```python
from build123d import *

# Parameters (mm, degrees)
BOSS_EXTRUDE1_DEPTH      = 38.1
CUT_EXTRUDE1_DEPTH       = 48.641761051
F_5_16_CLEARANCE_HOLE1_D = 8.3312
FILLET1_R                = 3.175
FILLET2_R                = 6.35


with BuildPart() as part:
    # Sketch1 → Boss-Extrude1 (new body)
    with BuildSketch(Plane.XY.offset(19.05)):
        with BuildLine():
            Line((0, 38.1), (0, 0))
            Line((0, 0), (14.986, 0))
            Line((14.986, 0), (14.986, -35.0266))
            ThreePointArc((14.986, -35.0266), (19.476128061, -33.166728061), (21.336, -28.6766))
            Line((21.336, -28.6766), (21.336, 6.35))
            Line((21.336, 6.35), (6.35, 6.35))
            Line((6.35, 6.35), (6.35, 31.75))
            ThreePointArc((6.35, 31.75), (4.490128061, 36.240128061), (0, 38.1))
        make_face()
    extrude(amount=-BOSS_EXTRUDE1_DEPTH)

    # Sketch2 → Cut-Extrude1 (cut, through all)
    with BuildSketch(Plane.ZY):
        with BuildLine():
            Line((-4.1656, 29.3624), (-4.1656, 16.6624))
            ThreePointArc((-4.1656, 16.6624), (0, 12.4968), (4.1656, 16.6624))
            Line((4.1656, 16.6624), (4.1656, 29.3624))
            ThreePointArc((4.1656, 29.3624), (0, 33.528), (-4.1656, 29.3624))
        make_face()
    extrude(amount=-CUT_EXTRUDE1_DEPTH, mode=Mode.SUBTRACT)

    # 5/16 Clearance Hole1 (through all)
    with Locations(Plane.ZY.offset(-14.986)):
        with Locations((0, -19.05)):
            Hole(F_5_16_CLEARANCE_HOLE1_D / 2)

    # Fillet1
    fillet1_edges = [part.edges().sort_by_distance(p)[0] for p in [
        (14.986, 0, 0),
    ]]
    fillet(fillet1_edges, radius=FILLET1_R)

    # Fillet2
    fillet2_edges = [part.edges().sort_by_distance(p)[0] for p in [
        (6.35, 6.35, 0),
        (21.336, 6.35, 0),
    ]]
    fillet(fillet2_edges, radius=FILLET2_R)


solid = part.part
```
Work out the finished part from the listing and answer in its coordinate system (mm). A direction names the side the tool comes from. Give positions to 0.01 mm unless a question says otherwise; leave off trailing zeros. Write each loop counter-clockwise with the first axis right and the second up, starting at its lowest first coordinate (ties: lowest second). Pieces come first, ordered by that corner, then holes.
(1) Which of the six approach directions +Z, -Z, +X, -X, +Y, -Y give full straight-line access (tool end or side, diameter ignored) to faces 1 (the flat face through (3, 23, 4.166)), 2 (the flat face through (6.35, 22, 12)), 3 (the flat face through (14.986, -19, 5))?
Final values:
face 1: +X, -X
face 2: +Z, -Z, +X, +Y
face 3: +Z, -Z, -X, -Y
(2) Straight lines are drawn through the part: line 1 (Z direction, x = 2.25, y = 22); line 2 (X direction, y = 18, z = -9.5); line 3 (Y direction, x = 20, z = 0). For each, find the intervals that lie inside material, in ascending order.
Final values:
line 1: z = -19.05 to -4.17, 4.17 to 19.05
line 2: x = 0 to 6.35
line 3: y = -32.57 to -23.22, -14.88 to 3.9
(3) The part is cut by section B-B on z = -9.5. Write down the section's boundary in (x, y) (3 decimals), plus the area to 3 significant figures.
Final values:
outline: (0, 0) - (11.811, 0) arc R3.175 cw to (14.986, -3.175) - (14.986, -35.027) arc R6.35 ccw to (21.336, -28.677) - (21.336, 0) arc R6.35 ccw to (14.986, 6.35) - (12.7, 6.35) arc R6.35 cw to (6.35, 12.7) - (6.35, 31.75) arc R6.35 ccw to (0, 38.1) - close
area: 544 mm2
(4) The mould has two halves that part along Z. Classify faces 4 (the flat face through (21.336, -14.5, 0.3)), 5 (the flat face through (3, 23, -4.166)): pulls with the +Z half, pulls with the -Z half, needs draft (parallel to the pull), parting line crosses it, or undercut.
Final values:
face 4: needs draft
face 5: undercut
(5) The part is cut by section C-C on z = 2. Write down the section's boundary in (x, y) (3 decimals).
Final values:
outline: (0, 0) - (11.811, 0) arc R3.175 cw to (14.986, -3.175) - (14.986, -15.396) - (21.336, -15.396) - (21.336, 0) arc R6.35 ccw to (14.986, 6.35) - (12.7, 6.35) arc R6.35 cw to (6.35, 12.7) - (6.35, 13.008) - (0, 13.008) - close; (0, 33.016) - (6.222, 33.016) arc R6.35 ccw to (0, 38.1) - close; (14.986, -35.027) arc R6.35 ccw to (21.336, -28.677) - (21.336, -22.704) - (14.986, -22.704) - close
(6) The part is cut by section A-A on y = -19.05. Write down the section's boundary in (x, z), plus the area to 3 significant figures.
Final values:
outline: (14.99, -19.05) - (21.34, -19.05) - (21.34, -4.17) - (14.99, -4.17) - close; (14.99, 4.17) - (21.34, 4.17) - (21.34, 19.05) - (14.99, 19.05) - close
area: 189 mm2
(7) Flat-ended cylindrical pins translate along their axes: pin 1 Ø1 at (x, z) = (14, 0.5) entering from +Y; pin 2 Ø14 at (y, z) = (26, -10.5) entering from +X; pin 3 Ø4 at (x, z) = (12.5, -4.5) entering from +Y. Find the tip coordinate at first contact, or state that the pin passes through.
Final values:
pin 1: stops at y = 6.35
pin 2: stops at x = 6.35
pin 3: stops at y = 6.74
(8) The part is cut by section D-D on x = 18.5. Write down the section's boundary in (y, z).
Final values:
outline: (-33.97, -19.05) - (5.29, -19.05) - (5.29, 19.05) - (-33.97, 19.05) - close; hole circle Ø8.33 at (-19.05, 0)
